Input: part model. Units: mm. Frame: model coordinates. Face numbers are marked on the shaded views. A direction names the side the tool comes from. Round coordinates to 2 decimals unless told otherwise and drop trailing zeros. Order: outer loops, then holes, each group sorted by start corner. A loop starts at its lowest first (then second) coordinate and runs counter-clockwise, first axis right, second up.
Item 1: Mould query, pull axis Y, two halves, no side actions, for the marked faces 1, 2, 3 and 4. Classes: released by +Y, released by -Y, zero draft, split by the parting line, or undercut.
Item 2: Line query: L1, parallel to X at y = -3.5, z = 1.5; L2, parallel to X at y = -12.5, z = 0.95. Output: solid intervals per line, ascending.
Item 3: First-contact query: pin 1 (12 mm diameter, centred on x = 9.5, y = -9.5, fed in from -Z). Flat tip, straight axial feed; report the tip coordinate or a pass-through.
Item 4: Reachability of the marked faces 5 and 6 from +Z, -Z, +X, -X, +Y, -Y: full face, straight path, thin tool, end or side. Return the list, or none.
Item 5: Cut plane A-A on x = 6. Output: boundary loops of the cut face in (y, z), then the cut area to 3 significant figures.
Item 6: Cut plane C-C on z = 1.2. Output: boundary loops of the cut face in (x, y), then the cut area to 3 significant figures.
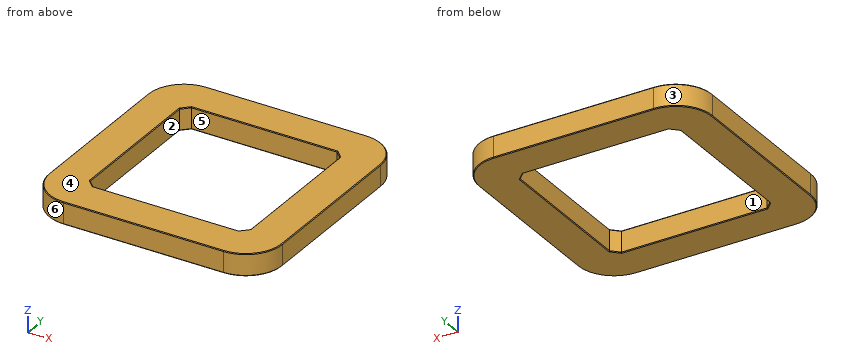
```python
from build123d import *

# Parameters (mm, degrees)
F0_W     = 32
F0_H     = 32
F0_W_2   = 22
F0_H_2   = 22
F1_DEPTH = 3
F2_SIZE2 = 1
F2_SIZE  = 1
F3_R     = 5
F4_SIZE  = 0.1


with BuildPart() as f1:
    # F0 (on Top) → F1 (new body)
    with BuildSketch(Plane.XY):
        Rectangle(F0_W, F0_H)
        Rectangle(F0_W_2, F0_H_2, mode=Mode.SUBTRACT)
    extrude(amount=F1_DEPTH)

    # F2
    f2_edges = [f1.edges().sort_by_distance(p)[0] for p in [
        (-11, 11, 1.5),
        (-11, -11, 1.5),
        (11, 11, 1.5),
        (11, -11, 1.5),
    ]]
    chamfer(f2_edges, length=F2_SIZE, length2=F2_SIZE2)

    # F3
    f3_edges = [f1.edges().sort_by_distance(p)[0] for p in [
        (16, 16, 1.5),
        (16, -16, 1.5),
        (-16, -16, 1.5),
        (-16, 16, 1.5),
    ]]
    fillet(f3_edges, radius=F3_R)

    # F4
    f4_edges = [f1.edges().sort_by_distance(p)[0] for p in [
        (0, 16, 3),
        (14.535534, 14.535534, 3),
        (-14.535534, 14.535534, 3),
        (16, 0, 3),
        (-16, 0, 3),
        (14.535534, -14.535534, 3),
        (-14.535534, -14.535534, 3),
        (0, -16, 3),
        (-11, 0, 3),
        (-10.5, -10.5, 3),
        (-10.5, 10.5, 3),
        (0, -11, 3),
        (0, 11, 3),
        (10.5, -10.5, 3),
        (10.5, 10.5, 3),
        (11, 0, 3),
        (0, 16, 0),
        (14.535534, 14.535534, 0),
        (-14.535534, 14.535534, 0),
        (16, 0, 0),
        (-16, 0, 0),
        (14.535534, -14.535534, 0),
        (-14.535534, -14.535534, 0),
        (0, -16, 0),
        (-11, 0, 0),
        (-10.5, -10.5, 0),
        (-10.5, 10.5, 0),
        (0, -11, 0),
        (0, 11, 0),
        (10.5, -10.5, 0),
        (10.5, 10.5, 0),
        (11, 0, 0),
    ]]
    chamfer(f4_edges, length=F4_SIZE)


solid = f1.part
```
From the geometry:
1. face 1: undercut
1. face 2: undercut
1. face 3: released by +Y
1. face 4: zero draft
2. L1: x = -16 to -11, 11 to 16
2. L2: x = -15.77 to 15.77
3. pin 1: stops at z = 0
4. face 5: +Z, -Z
4. face 6: +Z, -Z, -X, -Y
5. outline: (-16, 0.1) - (-15.9, 0) - (-11.1, 0) - (-11, 0.1) - (-11, 2.9) - (-11.1, 3) - (-15.9, 3) - (-16, 2.9) - close; (11, 0.1) - (11.1, 0) - (15.9, 0) - (16, 0.1) - (16, 2.9) - (15.9, 3) - (11.1, 3) - (11, 2.9) - close
5. area: 30.0 mm2
6. outline: (-16, -11) arc R5 ccw to (-11, -16) - (11, -16) arc R5 ccw to (16, -11) - (16, 11) arc R5 ccw to (11, 16) - (-11, 16) arc R5 ccw to (-16, 11) - close; hole (-11, -10) - (-10, -11) - (10, -11) - (11, -10) - (11, 10) - (10, 11) - (-10, 11) - (-11, 10) - close
6. area: 521 mm2
